from build123d import *

# Parameters (mm, degrees)
SKETCH3_W          = 16
SKETCH3_H          = 2
CHAMFER1_SIZE      = 0.6
CUT_EXTRUDE1_DEPTH = 1.61
SKETCH9_R          = 1.443375673
CUT_EXTRUDE2_DEPTH = 1.61
CUT_EXTRUDE2_DRAFT = -45


with BuildPart() as part:
    # Sketch3 → Revolve1 (revolve)
    with BuildSketch(Plane(origin=(0, 0, 0), x_dir=(0, 0, -1), z_dir=(1, 0, 0))):
        with Locations((0, 1)):
            Rectangle(SKETCH3_W, SKETCH3_H)
    revolve(axis=Axis((0, 0, -8), (0, 0, 1)))

    # Chamfer1
    chamfer1_edges = [part.edges().sort_by_distance(p)[0] for p in [
        (0, -2, -8),
    ]]
    chamfer(chamfer1_edges, length=CHAMFER1_SIZE)

    # Sketch6 → Revolve2 (revolve)
    with BuildSketch(Plane(origin=(0, 0, 0), x_dir=(0, 0, -1), z_dir=(1, 0, 0))):
        Polygon((-8, 4), (-7.7, 4), (-5.7, 2), (-5.7, 0), (-8, 0), align=None)
    revolve(axis=Axis((0, 0, -8), (0, 0, 1)))

    # Sketch8 → Cut-Extrude1 (cut)
    with BuildSketch(Plane.XY.offset(8)):
        Polygon((0, 1.443375673), (-1.25, 0.721687836), (-1.25, -0.721687836), (0, -1.443375673), (1.25, -0.721687836), (1.25, 0.721687836), align=None)
    extrude(amount=-CUT_EXTRUDE1_DEPTH, mode=Mode.SUBTRACT)


with BuildPart() as cut_extrude2_tool:
    # Sketch9 → Cut-Extrude2 (with draft: the straight prism first)
    with BuildSketch(Plane.XY.offset(8)):
        Circle(SKETCH9_R)
    extrude(amount=-CUT_EXTRUDE2_DEPTH)
    # Cut-Extrude2: the draft: its side faces are tilted about the plane it starts from
    cut_extrude2_sides = [cut_extrude2_tool.faces().sort_by_distance(p)[0] for p in [
        (-1.443375673, 0, 7.195),
    ]]
    draft(cut_extrude2_sides, Plane.XY.offset(8), CUT_EXTRUDE2_DRAFT)


with BuildPart() as part_1:
    add(part.part)

    # Cut-Extrude2: cut by cut_extrude2_tool
    add(cut_extrude2_tool.part, mode=Mode.SUBTRACT)


solid = part_1.part
Design review of the part built by this model. Coordinates are the model's own, in mm. A direction names the side the tool comes from. Coordinates: 2 decimals unless noted, no trailing zeros. Loops run counter-clockwise (first coordinate to the right, second up) from the corner with the lowest first, then second, coordinate; pieces in that order, holes last. Notation, with made-up numbers: (-30.75, 60) - (8.25, 60) arc R23 ccw to (8.25, 93) - close; hole circle Ø8 at (-18.5, 1.25). An arc over 180 degrees is marked (long way). Use CSV: the item, a comma, the result in double quotes. Start each with the question number.
1. Add section B-B on z = -0.5. Give the boundary of the cut face in (x, y), plus the area to 3 significant figures.
2. To check wall thickness, follow probe 1 along Z at (x, y) = (-0.25, -1.25); probe 2 along X at (y, z) = (-0.5, -7); probe 3 along Y at (x, z) = (0.25, 5). State the ranges of each line that lie inside material, in increasing order.
3. Add section C-C on z = 6. Give the boundary of the cut face in (x, y), plus the area to 3 significant figures.
4. Mouldability with a two-part tool opening along Y and no side actions: class faces 3 (the flat face through (0, -2, 8)), 4 (the cylindrical face through (2, 0, -1)), 5 (the flat face through (0.63, 1.08, 7.21)) as released by +Y, released by -Y, zero draft, split by the parting line, or undercut.
5. Clearance check with flat-ended pins moving along their axes: pin 1 (3 mm diameter, centred on y = -3, z = 3, fed in from +X); pin 2 (4 mm diameter, centred on y = -2, z = 1, fed in from +X); pin 3 (1.5 mm diameter, centred on y = 2.5, z = 3.5, fed in from -X). State where each tip first meets the part, or that it passes through.
6. For faces 1 (the flat face through (0, 0, -8)), 2 (the flat face through (0.616, -1.088, 7.206)), list the 3-axis set-ups (+Z, -Z, +X, -X, +Y, -Y) from which the entire face can be reached by the end or side of a thin tool; tool diameter is ignored.
7. Add section A-A on y = 0. Give the boundary of the cut face in (x, z).
Resolved:
1,outline,"circle Ø4 at (0, 0)"
1,area,"12.6 mm2"
2,probe 1,"-8 to 6.39"
2,probe 2,"-1.94 to 1.94"
2,probe 3,"-1.98 to 1.98"
3,outline,"circle Ø4.6 at (0, 0)"
3,area,"16.6 mm2"
4,face 3,"zero draft"
4,face 4,"split by the parting line"
4,face 5,"undercut"
5,pin 1,"x = 1.32"
5,pin 2,"x = 2"
5,pin 3,"x = -0.97"
6,face 1,"-Z, +X, -X, +Y, -Y"
6,face 2,"+Z"
7,outline,"(-4, 7.7) - (-2, 5.7) - (-2, -7.4) - (-1.4, -8) - (1.4, -8) - (2, -7.4) - (2, 5.7) - (4, 7.7) - (4, 8) - (1.44, 8) - (1.25, 7.81) - (1.25, 6.39) - (-1.25, 6.39) - (-1.25, 7.81) - (-1.44, 8) - (-4, 8) - close"
